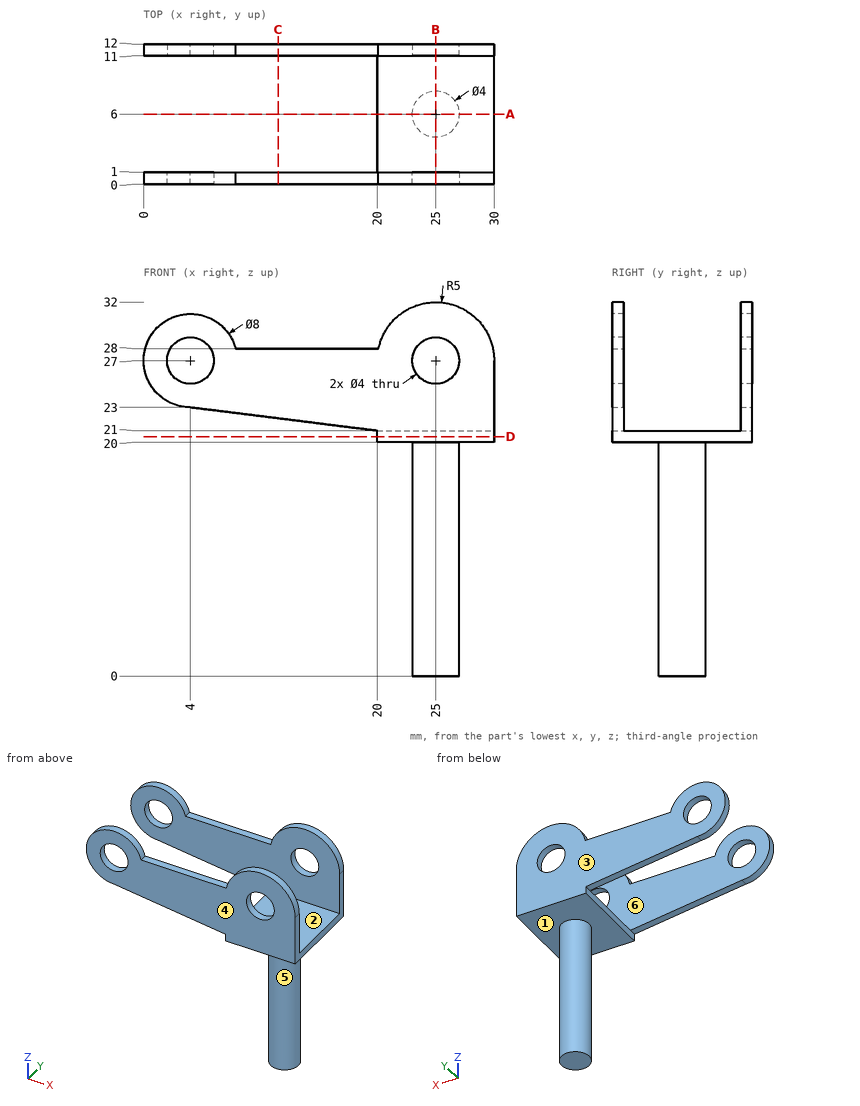
Geometry: see drawing. Coordinates: mm, zero at the bounding-box minimum. A direction names the side the tool comes from. Coordinates: 2 decimals unless noted, no trailing zeros. Loops run counter-clockwise (first coordinate to the right, second up) from the corner with the lowest first, then second, coordinate; pieces in that order, holes last. Notation, with made-up numbers: (53, 23) -> (74, 23) arc R15 cw to (74, 34) -> close; hole circle Ø2 at (52, 75). An arc over 180 degrees is marked (long way). Write item = value, one per line. Start each with the question number.
Item 1: Material intervals for line 1 (X direction, y = 11.55, z = 27); line 2 (Z direction, x = 25, y = 11.6); line 3 (Z direction, x = 4, y = 0.35), sorted ascending.
Item 2: Mould query, pull axis Y, two halves, no side actions, for the marked faces 4, 5 and 6. Classes: pulls with the +Y half, pulls with the -Y half, needs draft (parallel to the pull), parting line crosses it, or undercut.
Item 3: Cut plane C-C, the plane x = 11.5. Return loops of the section in (y, z), plus the area to 3 significant figures.
Item 4: Cut plane D-D, the plane z = 20.5. Return loops of the section in (x, y).
Item 5: Reachability of the marked faces 1, 2 and 3 from +Z, -Z, +X, -X, +Y, -Y: full face, straight path, thin tool, end or side. Return the list, or none.
Item 6: Cut plane B-B, the plane x = 25. Return loops of the section in (y, z).
Item 7: First-contact query: P1, Ø2.5, axis at x = 4, z = 27, coming from the +Y side; P2, Ø12, axis at x = 15.5, z = 17.5, coming from the +Y side; P3, Ø5, axis at y = 8.5, z = 15.5, coming from the -X side; P4, Ø0.8, axis at x = 11.5, y = 0.5, coming from the +Z side. Flat tips, straight axial feed; report the tip coordinate or a pass-through.
Item 8: Cut plane A-A, the plane y = 6. Return loops of the section in (x, z).
Ans:
q1.line_1 = 0 to 2, 6 to 23, 27 to 30
q1.line_2 = 20 to 25, 29 to 32
q1.line_3 = 23 to 25, 29 to 31
q2.face_4 = pulls with the -Y half
q2.face_5 = parting line crosses it
q2.face_6 = undercut
q3.outline = (0, 22.06) -> (1, 22.06) -> (1, 28) -> (0, 28) -> close; (11, 22.06) -> (12, 22.06) -> (12, 28) -> (11, 28) -> close
q3.area = 11.9 mm²
q4.outline = (20, 0) -> (30, 0) -> (30, 12) -> (20, 12) -> close
q5.face_1 = -Z
q5.face_2 = +Z, +X, -X
q5.face_3 = +Z, -Z, +X, -X, +Y
q6.outline = (0, 20) -> (4, 20) -> (4, 0) -> (8, 0) -> (8, 20) -> (12, 20) -> (12, 25) -> (11, 25) -> (11, 21) -> (1, 21) -> (1, 25) -> (0, 25) -> close; (0, 29) -> (1, 29) -> (1, 32) -> (0, 32) -> close; (11, 29) -> (12, 29) -> (12, 32) -> (11, 32) -> close
q7.P1 = through
q7.P2 = 12
q7.P3 = 23
q7.P4 = 28
q8.outline = (20, 20) -> (23, 20) -> (23, 0) -> (27, 0) -> (27, 20) -> (30, 20) -> (30, 21) -> (20, 21) -> close
